Here's how the part is built. I have some questions about the finished solid (model axes, mm). A direction names the side the tool comes from. Round coordinates to 2 decimals unless told otherwise and drop trailing zeros. Loops run counter-clockwise (first coordinate to the right, second up) from the corner with the lowest first, then second, coordinate; pieces in that order, holes last. Notation, with made-up numbers: M 62,50.25 L 83,50.25 A22 ccw 83,81.25 Z; hole C 81,-32 d9. An arc over 180 degrees is marked long. Use a Markdown table: item, result.
```python
from build123d import *

# Parameters (mm, degrees)
SKETCH_1_W          = 60
SKETCH_1_H          = 60
EXTRUDE_1_DEPTH     = 3
SKETCH_2_W          = 28
SKETCH_2_H          = 60
EXTRUDE_2_DEPTH     = 35
CUT_EXTRUDE_1_DEPTH = 60
SKETCH_4_R          = 12.5
CUT_EXTRUDE_2_DEPTH = 3
EXTRUDE_3_DEPTH     = 110
EXTRUDE_4_DEPTH     = 110
CUT_EXTRUDE_3_DEPTH = 100
CUT_EXTRUDE_5_DEPTH = 110
SKETCH_12_W         = 60
SKETCH_12_H         = 3
EXTRUDE_5_DEPTH     = 5
SKETCH_13_W         = 60
SKETCH_13_H         = 3
EXTRUDE_6_DEPTH     = 5


with BuildPart() as part:
    # 草图1 → 凸台-拉伸1 (new body)
    with BuildSketch(Plane.XY):
        with Locations((14.347634014, 11.597850928)):
            Rectangle(SKETCH_1_W, SKETCH_1_H)
    extrude(amount=EXTRUDE_1_DEPTH)

    # 草图2 → 凸台-拉伸2 (add)
    with BuildSketch(Plane(origin=(0, 0, 0), x_dir=(-1, 0, 0), z_dir=(0, 0, -1))):
        with Locations((-30.347634014, 11.597850928)):
            Rectangle(SKETCH_2_W, SKETCH_2_H)
        with Locations((1.652365986, 11.597850928)):
            Rectangle(SKETCH_2_W, SKETCH_2_H)
    extrude(amount=EXTRUDE_2_DEPTH)

    # 草图3 → 切除-拉伸1 (cut)
    with BuildSketch(Plane(origin=(0, 41.597850928, 0), x_dir=(1, 0, 0), z_dir=(0, 1, 0))):
        Polygon((16.347634014, 35), (44.347634014, 0), (44.347634014, 35), align=None)
        Polygon((12.347634014, 35), (-15.652365986, 0), (-15.652365986, 35), align=None)
    extrude(amount=-CUT_EXTRUDE_1_DEPTH, mode=Mode.SUBTRACT)

    # 草图4 → 切除-拉伸2 (cut)
    with BuildSketch(Plane.XY.offset(3)):
        with Locations((-1.652365986, 11.597850928)):
            Circle(SKETCH_4_R)
        with Locations((30.347634014, 11.597850928)):
            Circle(SKETCH_4_R)
    extrude(amount=-CUT_EXTRUDE_2_DEPTH, mode=Mode.SUBTRACT)

    # 草图5 → 凸台-拉伸3 (add)
    with BuildSketch(Plane(origin=(0, 41.597850928, 0), x_dir=(1, 0, 0), z_dir=(0, 1, 0))):
        Polygon((12.347634014, 35), (12.347634014, 0), (16.347634014, 0), (16.347634014, 20), (44.347634014, 0), (44.347634014, -3), (-15.652365986, -3), (-15.652365986, 0), align=None)
    extrude(amount=EXTRUDE_3_DEPTH)

    # 草图6 → 凸台-拉伸4 (add)
    with BuildSketch(Plane.XZ.offset(18.402149072)):
        Polygon((-15.652365986, 3), (-15.652365986, 0), (12.347634014, -35), (12.347634014, 0), (16.347634014, 0), (16.347634014, -35), (44.347634014, 0), (44.347634014, 3), align=None)
    extrude(amount=EXTRUDE_4_DEPTH)

    # 草图7 → 切除-拉伸3 (cut)
    with BuildSketch(Plane.XZ.offset(128.402149072)):
        Polygon((44.347634014, 0), (16.347634014, -35), (16.347634014, 0), align=None)
        Polygon((12.347634014, -35), (-15.652365986, 0), (12.347634014, 0), align=None)
    extrude(amount=-CUT_EXTRUDE_3_DEPTH, mode=Mode.SUBTRACT)

    # 草图9 → 切除-拉伸5 (cut)
    with BuildSketch(Plane(origin=(0, 151.597850928, 0), x_dir=(1, 0, 0), z_dir=(0, 1, 0))):
        Polygon((-15.652365986, 0), (12.347634014, 0), (12.347634014, 35), align=None)
        Polygon((16.347634014, 0), (44.347634014, 0), (16.347634014, 20), align=None)
    extrude(amount=-CUT_EXTRUDE_5_DEPTH, mode=Mode.SUBTRACT)

    # 草图12 → 凸台-拉伸5 (add)
    with BuildSketch(Plane(origin=(0, -128.402149072, 0), x_dir=(-1, 0, 0), z_dir=(0, -1, 0))):
        with Locations((-14.347634014, -1.5)):
            Rectangle(SKETCH_12_W, SKETCH_12_H)
    extrude(amount=EXTRUDE_5_DEPTH)

    # 草图13 → 凸台-拉伸6 (add)
    with BuildSketch(Plane(origin=(0, 151.597850928, 0), x_dir=(1, 0, 0), z_dir=(0, 1, 0))):
        with Locations((14.347634014, -1.5)):
            Rectangle(SKETCH_13_W, SKETCH_13_H)
    extrude(amount=EXTRUDE_6_DEPTH)


solid = part.part
```
Q1. Imagine slicing it at A-A, the plane z = -18. Please give me the cut outline in (x, y).
Return value:
| item | result |
|---|---|
| outline | M -1.25,-28.4 L 12.35,-28.4 L 12.35,41.6 L -1.25,41.6 Z; M 16.35,-28.4 L 29.95,-28.4 L 29.95,41.6 L 16.35,41.6 Z |
Q2. For faces 1 (the flat face through (30, 12, 0)), 2 (the flat face through (12.348, 7, -18)), 3 (the flat face through (24, -28.402, -9)), 4 (the flat face through (4, 41.598, -10)), which set-ups out of +Z, -Z, +X, -X, +Y, -Y let a thin tool reach every point of the face, with its end or its side?
Return value:
| item | result |
|---|---|
| face 1 | +Z |
| face 2 | -Z, +Y, -Y |
| face 3 | -Z, +X, -X, -Y |
| face 4 | -Z, +X, -X, +Y |
Q3. Imagine slicing it at D-D, the plane z = -3. Please give me the cut outline in (x, y), then the cut area to 3 significant figures.
Return value:
| item | result |
|---|---|
| outline | M -13.25,-28.4 L 12.35,-28.4 L 12.35,41.6 L -13.25,41.6 Z; M 16.35,-28.4 L 41.95,-28.4 L 41.95,41.6 L 16.35,41.6 Z |
| area | 3,580 mm^2 |
Q4. Imagine slicing it at C-C, the plane y = 124. Please give me the cut outline in (x, z), then the cut area to 3 significant figures.
Return value:
| item | result |
|---|---|
| outline | M -15.65,0 L 44.35,0 L 44.35,3 L -15.65,3 Z |
| area | 180 mm^2 |
Q5. Will these pins go through, and if not, where does the flat tip stop? P1, Ø2, axis at x = -8, y = -81.5, coming from the -Z side; P2, Ø8.5, axis at x = -1, z = -19.5, coming from the -Y side; P3, Ø14, axis at x = 0, z = -24.5, coming from the +Y side; P4, Ø8.5, axis at x = 35.5, z = -23.5, coming from the +Y side.
Return value:
| item | result |
|---|---|
| P1 | stops at z = 0 |
| P2 | stops at y = -28.4 |
| P3 | stops at y = 41.6 |
| P4 | passes through |
Q6. We'd pull the mould along X, two halves only. Please class faces 5 (the flat face through (2, -28.402, -13)), 6 (the flat face through (30.152, 7.088, -17.745)), 7 (the flat face through (16.348, 7, -17)): pulls with the +X half, pulls with the -X half, needs draft (parallel to the pull), parting line crosses it, or undercut.
Return value:
| item | result |
|---|---|
| face 5 | needs draft |
| face 6 | pulls with the +X half |
| face 7 | undercut |
Q7. Imagine slicing it at B-B, the plane x = 24. Please give me the cut outline in (y, z).
Return value:
| item | result |
|---|---|
| outline | M -133.4,0 L -28.4,0 L -28.4,-25.43 L 41.6,-25.43 L 41.6,0 L 156.6,0 L 156.6,3 L 22.37,3 L 22.37,0 L 0.83,0 L 0.83,3 L -133.4,3 Z |
Q8. I need wall thicknesses on line 1 (Z direction, x = 24, y = 46); line 2 (Y direction, x = 24, z = -2); line 3 (X direction, y = -25.5, z = -29.5). Which ranges of each line are inside material? Lowest first, please. Write a range as from..to.
Return value:
| item | result |
|---|---|
| line 1 | z = 0..3 |
| line 2 | y = -28.4..41.6 |
| line 3 | x = 7.95..12.35, 16.35..20.75 |
